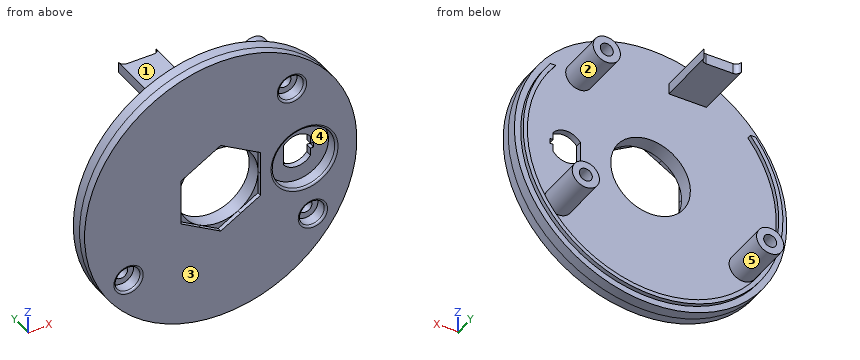
from build123d import *
from build123d.topology import SkipClean

# Parameters (mm, degrees)
SKETCH1_R           = 32.5
BOSS_EXTRUDE1_DEPTH = 21
SHELL1_T            = -2.5
CUT_EXTRUDE2_START  = -18.5
CUT_EXTRUDE2_DEPTH  = 18.5
BOSS_EXTRUDE2_DEPTH = 18.5
SKETCH9_R           = 3.25
BOSS_EXTRUDE3_DEPTH = 10.97
CUT_EXTRUDE4_START  = -18.5
CUT_EXTRUDE4_DEPTH  = 18.5
CUT_EXTRUDE5_DEPTH  = 70.707226983
BOSS_EXTRUDE4_DEPTH = 1
BOSS_EXTRUDE5_START = 2
SKETCH15_R          = 32.5
BOSS_EXTRUDE5_DEPTH = 2
SKETCH13_R          = 9.5
CUT_EXTRUDE6_DEPTH  = 49.052683588
CUT_EXTRUDE7_DEPTH  = 1
SKETCH18_R          = 7.5
CUT_EXTRUDE8_DEPTH  = 3
SKETCH21_R          = 3
CUT_EXTRUDE9_DEPTH  = 3
FILLET1_R           = 0.5
SKETCH23_R          = 1.55
CUT_EXTRUDE10_DEPTH = 49.51154914


with BuildPart() as part:
    # Sketch1 → Boss-Extrude1 (new body)
    with BuildSketch(Plane(origin=(0, 0, 0), x_dir=(1, 0, 0), z_dir=(0, 1, 0))):
        with Locations(Location((0, 0, 0), (0, 0, 90))):
            Circle(SKETCH1_R)
    extrude(amount=BOSS_EXTRUDE1_DEPTH)

    # Shell1
    shell1_openings = [part.faces().sort_by_distance(p)[0] for p in [
        (0, 21, 0),
    ]]
    offset(amount=SHELL1_T, openings=shell1_openings, kind=Kind.INTERSECTION)

    # Sketch4 → Cut-Extrude2 (cut)
    with BuildSketch(Plane(origin=(0, 21, 0), x_dir=(1, 0, 0), z_dir=(0, 1, 0)).offset(CUT_EXTRUDE2_START)):
        with BuildLine():
            Line((-19.2835, -22.981440942), (19.2835, -22.981440942))
            Line((19.2835, -22.981440942), (22.980499826, -22.981440942))
            ThreePointArc((22.980499826, -22.981440942), (0, -32.5), (-22.980499826, -22.981440942))
            Line((-22.980499826, -22.981440942), (-19.2835, -22.981440942))
        make_face()
    extrude(amount=CUT_EXTRUDE2_DEPTH, mode=Mode.SUBTRACT)

    # Sketch5 → Boss-Extrude2 (add, through all)
    with SkipClean():  # the faces are left unmerged after this step: merging them gives an invalid solid
        with BuildSketch(Plane(origin=(0, 2.5, 0), x_dir=(1, 0, 0), z_dir=(0, 1, 0))):
            with BuildLine():
                Line((-22.980499826, -22.981440942), (22.980499826, -22.981440942))
                ThreePointArc((22.980499826, -22.981440942), (21.612881002, -24.27206985), (20.17290677, -25.481440942))
                Line((20.17290677, -25.481440942), (-20.17290677, -25.481440942))
                ThreePointArc((-20.17290677, -25.481440942), (-21.612881002, -24.27206985), (-22.980499826, -22.981440942))
            make_face()
        extrude(amount=BOSS_EXTRUDE2_DEPTH)

    # Sketch9 → Boss-Extrude3 (add)
    with SkipClean():  # the faces are left unmerged after this step: merging them gives an invalid solid
        with BuildSketch(Plane(origin=(0, 2.5, 0), x_dir=(1, 0, 0), z_dir=(0, 1, 0))):
            with Locations(Location((-22, 15, 0), (0, 0, 90))):
                Circle(SKETCH9_R)
            with Locations(Location((22, 15, 0), (0, 0, 90))):
                Circle(SKETCH9_R)
            with Locations(Location((17, -19, 0), (0, 0, 90))):
                Circle(SKETCH9_R)
        extrude(amount=BOSS_EXTRUDE3_DEPTH)

    # Sketch10 → Cut-Extrude4 (cut)
    with BuildSketch(Plane(origin=(0, 21, 0), x_dir=(1, 0, 0), z_dir=(0, 1, 0)).offset(CUT_EXTRUDE4_START)):
        with BuildLine():
            Line((-20.17290677, -25.481440942), (-13.33, -25.481440942))
            Line((-13.33, -25.481440942), (-13.33, -22.981440942))
            Line((-13.33, -22.981440942), (-19.2835, -22.981440942))
            ThreePointArc((-19.2835, -22.981440942), (0, 30), (19.2835, -22.981440942))
            Line((19.2835, -22.981440942), (-4.35, -22.981440942))
            Line((-4.35, -22.981440942), (-4.35, -25.481440942))
            Line((-4.35, -25.481440942), (20.17290677, -25.481440942))
            ThreePointArc((20.17290677, -25.481440942), (0, 32.5), (-20.17290677, -25.481440942))
        make_face()
    extrude(amount=CUT_EXTRUDE4_DEPTH, mode=Mode.SUBTRACT)

    # Sketch11 → Cut-Extrude5 (cut, through all)
    with BuildSketch(Plane.XY.offset(25.481440942)):
        with BuildLine():
            Line((-12.04, 15.23), (-5.64, 15.23))
            ThreePointArc((-5.64, 15.23), (-4.727832252, 15.607832252), (-4.35, 16.52))
            Line((-4.35, 16.52), (-4.35, 21))
            Line((-4.35, 21), (-13.33, 21))
            Line((-13.33, 21), (-13.33, 16.52))
            ThreePointArc((-13.33, 16.52), (-12.952167748, 15.607832252), (-12.04, 15.23))
        make_face()
    extrude(amount=-CUT_EXTRUDE5_DEPTH, mode=Mode.SUBTRACT)

    # Sketch12 → Boss-Extrude4 (add)
    with BuildSketch(Plane(origin=(0, 2.5, 0), x_dir=(1, 0, 0), z_dir=(0, 1, 0))):
        with BuildLine():
            Line((-24.509281911, -18.981440942), (-23.231549664, -18.981440942))
            ThreePointArc((-23.231549664, -18.981440942), (0, 30), (23.231549664, -18.981440942))
            Line((23.231549664, -18.981440942), (24.509281911, -18.981440942))
            ThreePointArc((24.509281911, -18.981440942), (0, 31), (-24.509281911, -18.981440942))
        make_face()
    extrude(amount=BOSS_EXTRUDE4_DEPTH)

    # Sketch15 → Boss-Extrude5 (add)
    with BuildSketch(Plane.XZ.offset(BOSS_EXTRUDE5_START)):
        with Locations(Location((0, 0, 0), (0, 0, 270))):
            Circle(SKETCH15_R)
    extrude(amount=-BOSS_EXTRUDE5_DEPTH)

    # Sketch13 → Cut-Extrude6 (cut, through all)
    with BuildSketch(Plane(origin=(0, 2.5, 0), x_dir=(1, 0, 0), z_dir=(0, 1, 0))):
        with Locations(Location((0, 0, 0), (0, 0, 270))):
            Circle(SKETCH13_R)
        with BuildLine():
            Line((16.775, 2.408318916), (16.775, -2.408318916))
            ThreePointArc((16.775, -2.408318916), (20, -4.025), (23.225, -2.408318916))
            Line((23.225, -2.408318916), (23.225, -0.625))
            Line((23.225, -0.625), (23.95, -0.625))
            Line((23.95, -0.625), (23.95, 0.625))
            Line((23.95, 0.625), (23.225, 0.625))
            Line((23.225, 0.625), (23.225, 2.408318916))
            ThreePointArc((23.225, 2.408318916), (20, 4.025), (16.775, 2.408318916))
        make_face()
    extrude(amount=-CUT_EXTRUDE6_DEPTH, mode=Mode.SUBTRACT)

    # Sketch17 → Cut-Extrude7 (cut)
    with BuildSketch(Plane.XZ.offset(2)):
        Polygon((9.5, -5.484827557), (9.5, 5.484827557), (0, 10.969655115), (-9.5, 5.484827557), (-9.5, -5.484827557), (0, -10.969655115), align=None)
    extrude(amount=-CUT_EXTRUDE7_DEPTH, mode=Mode.SUBTRACT)

    # Sketch18 → Cut-Extrude8 (cut)
    with BuildSketch(Plane.XZ.offset(2)):
        with Locations(Location((20, 0, 0), (0, 0, 270))):
            Circle(SKETCH18_R)
    extrude(amount=-CUT_EXTRUDE8_DEPTH, mode=Mode.SUBTRACT)

    # Sketch21 → Cut-Extrude9 (cut)
    with BuildSketch(Plane.XZ.offset(2)):
        with Locations(Location((-22, -15, 0), (0, 0, 270))):
            Circle(SKETCH21_R)
        with Locations(Location((22, -15, 0), (0, 0, 270))):
            Circle(SKETCH21_R)
        with Locations(Location((17, 19, 0), (0, 0, 270))):
            Circle(SKETCH21_R)
    extrude(amount=-CUT_EXTRUDE9_DEPTH, mode=Mode.SUBTRACT)

    # Fillet1
    fillet1_edges = [part.edges().sort_by_distance(p)[0] for p in [
        (20, -2, 7.5),
        (-22, -2, -12),
        (22, -2, -12),
        (17, -2, 22),
    ]]
    fillet(fillet1_edges, radius=FILLET1_R)

    # Sketch23 → Cut-Extrude10 (cut, through all)
    with BuildSketch(Plane.XZ.offset(-1)):
        with Locations(Location((-22, -15, 0), (0, 0, 270))):
            Circle(SKETCH23_R)
        with Locations(Location((17, 19, 0), (0, 0, 270))):
            Circle(SKETCH23_R)
        with Locations(Location((22, -15, 0), (0, 0, 270))):
            Circle(SKETCH23_R)
    extrude(amount=-CUT_EXTRUDE10_DEPTH, mode=Mode.SUBTRACT)


solid = part.part
Can you work these out from the model? Positions are in its coordinate system, mm. Face numbers are marked on the shaded views. A direction names the side the tool comes from. Give positions to 0.01 mm unless a question says otherwise; leave off trailing zeros. Order: outer loops, then holes, each group sorted by start corner. A loop starts at its lowest first (then second) coordinate and runs counter-clockwise, first axis right, second up. Notation, with made-up numbers: M 21,-30 L 34,-30 A19 cw 34,0 Z; hole C 36.25,-17 d11. An arc over 180 degrees is marked long. Use a Markdown table: item, result. Add a question column.
Item 1: Suppose I cut it at B-B (x = -22). List the corners of the cut face in (y, z) for me, then the cut area to 3 significant figures.
Item 2: Suppose I cut it at D-D (x = -1). List the corners of the cut face in (y, z) for me.
Item 3: Suppose I cut it at A-A (y = 5). List the corners of the cut face in (x, z) for me, then the cut area to 3 significant figures.
Item 4: Suppose I cut it at C-C (z = 1.5). Count the separate pieces of the cut face and the enclosed holes in it, then the cut area to 3 significant figures.
Item 5: We'd pull the mould along Z, two halves only. Please class the marked faces 1, 2 and 3: +Z half, -Z half, draft (parallel to the pull), parting line (faces both ways), or undercut.
Item 6: For the marked faces 4 and 5, which set-ups out of +Z, -Z, +X, -X, +Y, -Y let a thin tool reach every point of the face, with its end or its side?
Item 7: Will these pins go through, and if not, where does the flat tip stop? pin 1 (3 mm diameter, centred on x = 15.5, y = 13.5, fed in from -Z); pin 2 (0.8 mm diameter, centred on x = -24, y = 3, fed in from +Z); pin 3 (3.5 mm diameter, centred on x = -22, z = -15, fed in from -Y).
Item 8: If I drill on L1, parallel to X at y = 7, z = -15; L2, parallel to X at y = 9, z = 19; L3, parallel to X at y = 0.1, z = 0, over which ranges is the centre line in solid material (lowest first)? Write a range as [from, to].
Answer sheet:
| question | item | result |
|---|---|---|
| 1 | outline | M -2,-23.92 L 2.5,-23.92 L 2.5,-21.84 L 3.5,-21.84 L 3.5,-20.4 L 2.5,-20.4 L 2.5,-18.25 L 13.47,-18.25 L 13.47,-16.55 L 1,-16.55 L 1,-18 L -1.5,-18 A0.5 ccw -2,-18.5 Z; M -2,-11.5 A0.5 ccw -1.5,-12 L 1,-12 L 1,-13.45 L 13.47,-13.45 L 13.47,-11.75 L 2.5,-11.75 L 2.5,23.92 L -2,23.92 Z |
| 1 | area | 231 mm² |
| 2 | outline | M -2,-32.48 L 2.5,-32.48 L 2.5,-30.98 L 3.5,-30.98 L 3.5,-29.98 L 2.5,-29.98 L 2.5,-9.45 L -1,-9.45 L -1,-10.39 L -2,-10.39 Z; M -2,10.39 L -1,10.39 L -1,9.45 L 2.5,9.45 L 2.5,32.48 L -2,32.48 Z |
| 3 | outline | C -22,-15 d6.5; M -13.33,22.98 L -4.35,22.98 L -4.35,25.48 L -13.33,25.48 Z; C 17,19 d6.5; C 22,-15 d6.5; hole C -22,-15 d3.1; hole C 17,19 d3.1; hole C 22,-15 d3.1 |
| 3 | area | 99.4 mm² |
| 4 | separate pieces | 3 |
| 4 | enclosed holes | 0 |
| 4 | area | 156 mm² |
| 5 | face 1 | +Z half |
| 5 | face 2 | undercut |
| 5 | face 3 | draft |
| 6 | face 4 | -Y |
| 6 | face 5 | +Y |
| 7 | pin 1 | stops at z = 15.75 |
| 7 | pin 2 | stops at z = 18.98 |
| 7 | pin 3 | stops at y = 1 |
| 8 | L1 | x = [-25.25, -23.55], [-20.45, -18.75], [18.75, 20.45], [23.55, 25.25] |
| 8 | L2 | x = [13.75, 15.45], [18.55, 20.25] |
| 8 | L3 | x = [-32.5, -9.5], [9.5, 12.5], [27.5, 32.5] |
